Here's how the part is built. I have some questions about the finished solid (model axes, mm). A direction names the side the tool comes from. Give positions to 0.01 mm unless a question says otherwise; leave off trailing zeros. Order: outer loops, then holes, each group sorted by start corner. A loop starts at its lowest first (then second) coordinate and runs counter-clockwise, first axis right, second up. Notation, with made-up numbers: M -39.5,-29 L -27.5,-29 A9 ccw -27.5,-20 Z; hole C 2,77 d8. An arc over 180 degrees is marked long. Use one line per item in the form item = value.
from build123d import *

# Parameters (mm, degrees)
F1_DEPTH = 2.5
F3_DEPTH = 25.4
F4_R     = 29.845
F5_DEPTH = 25.4
F6_R     = 2.54
F7_DEPTH = 25.4
F8_R     = 5.08


with BuildPart() as f1:
    # F0 (on Front) → F1 (new body)
    with BuildSketch(Plane.XZ):
        with BuildLine():
            ThreePointArc((90.17, 79.375), (88.3101280605, 83.8651280605), (83.82, 85.725))
            Line((83.82, 85.725), (-83.82, 85.725))
            ThreePointArc((-83.82, 85.725), (-88.3101280605, 83.8651280605), (-90.17, 79.375))
            Line((-90.17, 79.375), (-90.17, -79.375))
            ThreePointArc((-90.17, -79.375), (-88.3101280605, -83.8651280605), (-83.82, -85.725))
            Line((-83.82, -85.725), (83.82, -85.725))
            ThreePointArc((83.82, -85.725), (88.3101280605, -83.8651280605), (90.17, -79.375))
            Line((90.17, -79.375), (90.17, 79.375))
        make_face()
    extrude(amount=F1_DEPTH)

    # F2 (on face) → F3 (cut)
    with BuildSketch(Plane.XZ.offset(2.5)):
        with BuildLine():
            Line((51.435, 24.765), (24.765, 24.765))
            ThreePointArc((24.765, 24.765), (22.5199359697, 23.8350640303), (21.59, 21.59))
            Line((21.59, 21.59), (21.59, -33.02))
            ThreePointArc((21.59, -33.02), (22.5199359697, -35.2650640303), (24.765, -36.195))
            Line((24.765, -36.195), (51.435, -36.195))
            ThreePointArc((51.435, -36.195), (53.6800640303, -35.2650640303), (54.61, -33.02))
            Line((54.61, -33.02), (54.61, 21.59))
            ThreePointArc((54.61, 21.59), (53.6800640303, 23.8350640303), (51.435, 24.765))
        make_face()
    extrude(amount=-F3_DEPTH, mode=Mode.SUBTRACT)

    # F4 (on face) → F5 (cut)
    with BuildSketch(Plane.XZ.offset(2.5)):
        with BuildLine():
            ThreePointArc((-14.605, 23.0316061483), (-10.8232361729, 30.9808186575), (-9.525, 39.6875))
            ThreePointArc((-9.525, 39.6875), (-10.8232361729, 48.3941813425), (-14.605, 56.3433938517))
            Line((-14.605, 56.3433938517), (-14.605, 23.0316061483))
        make_face()
        with BuildLine():
            Line((-14.605, 23.0316061483), (-14.605, 56.3433938517))
            ThreePointArc((-14.605, 56.3433938517), (-18.2663981155, 60.7911018845), (-22.7141061483, 64.4525))
            Line((-22.7141061483, 64.4525), (-56.0258938517, 64.4525))
            ThreePointArc((-56.0258938517, 64.4525), (-60.4736018845, 60.7911018845), (-64.135, 56.3433938517))
            Line((-64.135, 56.3433938517), (-64.135, 23.0316061483))
            ThreePointArc((-64.135, 23.0316061483), (-60.4736018845, 18.5838981155), (-56.0258938517, 14.9225))
            Line((-56.0258938517, 14.9225), (-22.7141061483, 14.9225))
            ThreePointArc((-22.7141061483, 14.9225), (-18.2663981155, 18.5838981155), (-14.605, 23.0316061483))
        make_face()
        with BuildLine():
            ThreePointArc((-22.7141061483, 64.4525), (-18.2663981155, 60.7911018845), (-14.605, 56.3433938517))
            Line((-14.605, 56.3433938517), (-14.605, 64.4525))
            Line((-14.605, 64.4525), (-22.7141061483, 64.4525))
        make_face()
        with BuildLine():
            Line((-14.605, 14.9225), (-14.605, 23.0316061483))
            ThreePointArc((-14.605, 23.0316061483), (-18.2663981155, 18.5838981155), (-22.7141061483, 14.9225))
            Line((-22.7141061483, 14.9225), (-14.605, 14.9225))
        make_face()
        with BuildLine():
            Line((-56.0258938517, 64.4525), (-22.7141061483, 64.4525))
            ThreePointArc((-22.7141061483, 64.4525), (-39.37, 69.5325), (-56.0258938517, 64.4525))
        make_face()
        with BuildLine():
            ThreePointArc((-56.0258938517, 14.9225), (-39.37, 9.8425), (-22.7141061483, 14.9225))
            Line((-22.7141061483, 14.9225), (-56.0258938517, 14.9225))
        make_face()
        with BuildLine():
            ThreePointArc((-64.135, 56.3433938517), (-60.4736018845, 60.7911018845), (-56.0258938517, 64.4525))
            Line((-56.0258938517, 64.4525), (-64.135, 64.4525))
            Line((-64.135, 64.4525), (-64.135, 56.3433938517))
        make_face()
        with BuildLine():
            Line((-64.135, 14.9225), (-56.0258938517, 14.9225))
            ThreePointArc((-56.0258938517, 14.9225), (-60.4736018845, 18.5838981155), (-64.135, 23.0316061483))
            Line((-64.135, 23.0316061483), (-64.135, 14.9225))
        make_face()
        with BuildLine():
            Line((-64.135, 23.0316061483), (-64.135, 56.3433938517))
            ThreePointArc((-64.135, 56.3433938517), (-69.215, 39.6875), (-64.135, 23.0316061483))
        make_face()
        with Locations((-39.37, -39.6875)):
            Circle(F4_R)
    extrude(amount=-F5_DEPTH, mode=Mode.SUBTRACT)

    # F6 (on face) → F7 (cut)
    with BuildSketch(Plane.XZ.offset(2.5)):
        with Locations((-82.55, 78.105)):
            Circle(F6_R)
        with Locations((82.55, 78.105)):
            Circle(F6_R)
        with Locations((82.55, -78.105)):
            Circle(F6_R)
        with Locations((-82.55, -78.105)):
            Circle(F6_R)
    extrude(amount=-F7_DEPTH, mode=Mode.SUBTRACT)

    # F8
    f8_edges = [f1.edges().sort_by_distance(p)[0] for p in [
        (-64.135, -1.25, 14.9225),
        (-14.605, -1.25, 14.9225),
        (-14.605, -1.25, 64.4525),
        (-64.135, -1.25, 64.4525),
    ]]
    fillet(f8_edges, radius=F8_R)


solid = f1.part
Q1. I want a section at A-A on x = -39.37. Write out the boundary of the cut face in (y, z) (1 decimal), then the cut area to 3 significant figures.
Found:
outline = M -2.5,-85.7 L 0,-85.7 L 0,-69.5 L -2.5,-69.5 Z; M -2.5,-9.8 L 0,-9.8 L 0,9.8 L -2.5,9.8 Z; M -2.5,69.5 L 0,69.5 L 0,85.7 L -2.5,85.7 Z
area = 130 mm²
Q2. I want a section at C-C on z = 12. Write out the boundary of the cut face in (x, y), then the cut area to 3 significant figures.
Found:
outline = M -90.17,-2.5 L -50.51,-2.5 L -50.51,0 L -90.17,0 Z; M -28.23,-2.5 L 21.59,-2.5 L 21.59,0 L -28.23,0 Z; M 54.61,-2.5 L 90.17,-2.5 L 90.17,0 L 54.61,0 Z
area = 313 mm²
Q3. Thinking about a two-plate mould opening in Z: for faces 3 (the face through (-39.12, -1.27, 69.53)), 4 (the face through (81.999, -1.268, -80.585)), 5 (the face through (19, -2.5, 1)), 6 (the face through (88.26, -1.232, -83.914)), which applies, +Z half, -Z half, draft (parallel to the pull), parting line (faces both ways), or undercut?
Found:
face_3 = undercut
face_4 = undercut
face_5 = draft
face_6 = -Z half
Q4. I want a section at B-B on z = -48. Write out the boundary of the cut face in (x, y), then the cut area to 3 significant figures.
Found:
outline = M -90.17,-2.5 L -68.03,-2.5 L -68.03,0 L -90.17,0 Z; M -10.71,-2.5 L 90.17,-2.5 L 90.17,0 L -10.71,0 Z
area = 308 mm²
Q5. I need wall thicknesses on L1, parallel to X at y = -0.6, z = 78; L2, parallel to Z at x = 82.55, y = -0.6 (3 decimals); L3, parallel to Z at x = 45, y = -1.3 (3 decimals). Which ranges of each line are inside material? Lowest first, please.
Found:
L1 = -90.17 to -85.09, -80.01 to 80.01, 85.09 to 90.17
L2 = -85.725 to -80.645, -75.565 to 75.565, 80.645 to 85.725
L3 = -85.725 to -36.195, 24.765 to 85.725
Q6. I want a section at D-D on y = -2. State how many separate pieces and enclosed holes the cut face has, then the cut area to 3 significant figures.
Found:
separate_pieces = 1
enclosed_holes = 7
area = 23,100 mm²
Q7. On a 3-axis mill with a long thin cutter (end or side, diameter ignored), from which of +Z, -Z, +X, -X, +Y, -Y can I reach the whole of each face in a straight line? I mean faces 1 (the face through (-88.359, -1.232, -83.815)), 2 (the face through (-62.61, -1.23, 63)). Say none if no direction works.
Found:
face_1 = -Z, -X, +Y, -Y
face_2 = +Y, -Y
Q8. I'm going to push a flat-ended pin straight in: pin 1 Ø3 at (x, z) = (82.55, 78.105) entering from +Y. Where does the tip first touch, or does it pass through?
Found:
pin_1 = through
